Could you check a few things on this model? Use its own coordinates, in mm. Face numbers are marked on the shaded views. A direction names the side the tool comes from. Round coordinates to 2 decimals unless told otherwise and drop trailing zeros. Loops run counter-clockwise (first coordinate to the right, second up) from the corner with the lowest first, then second, coordinate; pieces in that order, holes last. Notation, with made-up numbers: (60, -11) - (102, -11) arc R25 ccw to (102, 24) - close; hole circle Ø7 at (-14.75, 8). An arc over 180 degrees is marked (long way). Use one line per item in the form item = value.
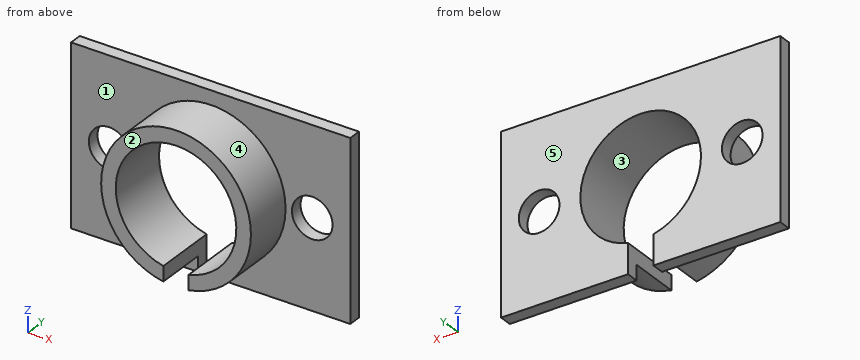
```python
from build123d import *

# Parameters (mm, degrees)
SKETCH_1_W          = 22
SKETCH_1_H          = 14
EXTRUDE_1_DEPTH     = 1
SKETCH_2_R          = 4.75
CUT_EXTRUDE_1_DEPTH = 14.076696831
SKETCH_3_R          = 5.9
SKETCH_3_R_2        = 4.75
EXTRUDE_2_DEPTH     = 4
SKETCH_4_R          = 1.6
CUT_EXTRUDE_2_DEPTH = 1
SKETCH_5_W          = 2
SKETCH_5_H          = 7.900772946
CUT_EXTRUDE_3_DEPTH = 10


with BuildPart() as part:
    # 草图1 → 凸台-拉伸1 (new body)
    with BuildSketch(Plane(origin=(0, 0, 0), x_dir=(1, 0, 0), z_dir=(0, 1, 0))):
        Rectangle(SKETCH_1_W, SKETCH_1_H)
    extrude(amount=EXTRUDE_1_DEPTH)

    # 草图2 → 切除-拉伸1 (cut, through all)
    with BuildSketch(Plane(origin=(0, 1, 0), x_dir=(1, 0, 0), z_dir=(0, 1, 0))):
        with Locations(Location((0, 0, 0), (0, 0, 270))):
            Circle(SKETCH_2_R)
    extrude(amount=-CUT_EXTRUDE_1_DEPTH, mode=Mode.SUBTRACT)

    # 草图3 → 凸台-拉伸2 (add)
    with BuildSketch(Plane(origin=(0, 0, 0), x_dir=(-1, 0, 0), z_dir=(0, -1, 0))):
        with Locations(Location((0, 0, 0), (0, 0, 270))):
            Circle(SKETCH_3_R)
        with Locations(Location((0, 0, 0), (0, 0, 270))):
            Circle(SKETCH_3_R_2, mode=Mode.SUBTRACT)
    extrude(amount=EXTRUDE_2_DEPTH)

    # 草图4 → 切除-拉伸2 (cut)
    with BuildSketch(Plane(origin=(0, 1, 0), x_dir=(1, 0, 0), z_dir=(0, 1, 0))):
        with Locations(Location((8, 0, 0), (0, 0, 270))):
            Circle(SKETCH_4_R)
        with Locations(Location((-8, 0, 0), (0, 0, 270))):
            Circle(SKETCH_4_R)
    extrude(amount=-CUT_EXTRUDE_2_DEPTH, mode=Mode.SUBTRACT)

    # 草图5 → 切除-拉伸3 (cut)
    with BuildSketch(Plane(origin=(0, 1, 0), x_dir=(1, 0, 0), z_dir=(0, 1, 0))):
        with Locations((0, 3.95882741)):
            Rectangle(SKETCH_5_W, SKETCH_5_H)
    extrude(amount=-CUT_EXTRUDE_3_DEPTH, mode=Mode.SUBTRACT)


solid = part.part
```
1. If we section it at B-B, the plane z = 0: Write out the boundary of the cut face in (x, y), plus the area to 3 significant figures.
Solution:
outline = (-11, 0) - (-9.6, 0) - (-9.6, 1) - (-11, 1) - close; (-6.4, 0) - (-5.9, 0) - (-5.9, -4) - (-4.75, -4) - (-4.75, 1) - (-6.4, 1) - close; (4.75, -4) - (5.9, -4) - (5.9, 0) - (6.4, 0) - (6.4, 1) - (4.75, 1) - close; (9.6, 0) - (11, 0) - (11, 1) - (9.6, 1) - close
area = 15.3 mm^2
2. If we section it at D-D, the plane z = 3.75: Write out the boundary of the cut face in (x, y).
Solution:
outline = (-11, 0) - (-4.55, 0) - (-4.55, -4) - (-2.92, -4) - (-2.92, 1) - (-11, 1) - close; (2.92, -4) - (4.55, -4) - (4.55, 0) - (11, 0) - (11, 1) - (2.92, 1) - close
3. For P1, Ø3, axis at y = -3, z = 0, coming from the +X side; P2, Ø1.2, axis at y = -2.5, z = -5.5, coming from the +X side; P3, Ø1.5, axis at y = -2.5, z = -3, coming from the +X side, each with a flat end and sliding along its axis, tell me the tip position at first contact or that it passes through.
Solution:
P1 = 5.9
P2 = 3.29
P3 = 5.45
4. Please list where these lines run through material, in increasing order: line 1 along X through (y, z) = (0.2, 0); line 2 along X through (y, z) = (-1.8, 0); line 3 along X through (y, z) = (0.4, -4.75).
Solution:
line_1 = -11 to -9.6, -6.4 to -4.75, 4.75 to 6.4, 9.6 to 11
line_2 = -5.9 to -4.75, 4.75 to 5.9
line_3 = -11 to -1, 1 to 11
5. On a 3-axis mill with a long thin cutter (end or side, diameter ignored), from which of +Z, -Z, +X, -X, +Y, -Y can I reach the whole of each face in a straight line? I mean the marked faces 1 and 2. Say none if no direction works.
Solution:
face_1 = -Y
face_2 = +Z, -Z, +X, -X, -Y
6. We'd pull the mould along Z, two halves only. Please class the marked faces 3, 4 and 5: +Z half, -Z half, draft (parallel to the pull), parting line (faces both ways), or undercut.
Solution:
face_3 = undercut
face_4 = parting line
face_5 = draft
7. If we section it at A-A, the plane x = 8: Write out the boundary of the cut face in (y, z), plus the area to 3 significant figures.
Solution:
outline = (0, -7) - (1, -7) - (1, -1.6) - (0, -1.6) - close; (0, 1.6) - (1, 1.6) - (1, 7) - (0, 7) - close
area = 10.8 mm^2
8. If we section it at C-C, the plane y = 0.5: Write out the boundary of the cut face in (x, z).
Solution:
outline = (-11, -7) - (-1, -7) - (-1, -4.64) arc R4.75 cw (long way) to (1, -4.64) - (1, -7) - (11, -7) - (11, 7) - (-11, 7) - close; hole circle Ø3.2 at (-8, 0); hole circle Ø3.2 at (8, 0)
